Part print with two shaded views. Sizes in mm from the minimum x, y, z corner. Give positions to 0.01 mm unless a question says otherwise; leave off trailing zeros. Order: outer loops, then holes, each group sorted by start corner. A loop starts at its lowest first (then second) coordinate and runs counter-clockwise, first axis right, second up. Notation, with made-up numbers: (5, 17.25) - (14, 17.25) arc R31 cw to (14, 50.25) - close; hole circle Ø7 at (51.25, 46.5). An arc over 180 degrees is marked (long way). Return JSON: item names as keys, results as strings. Group by question number.
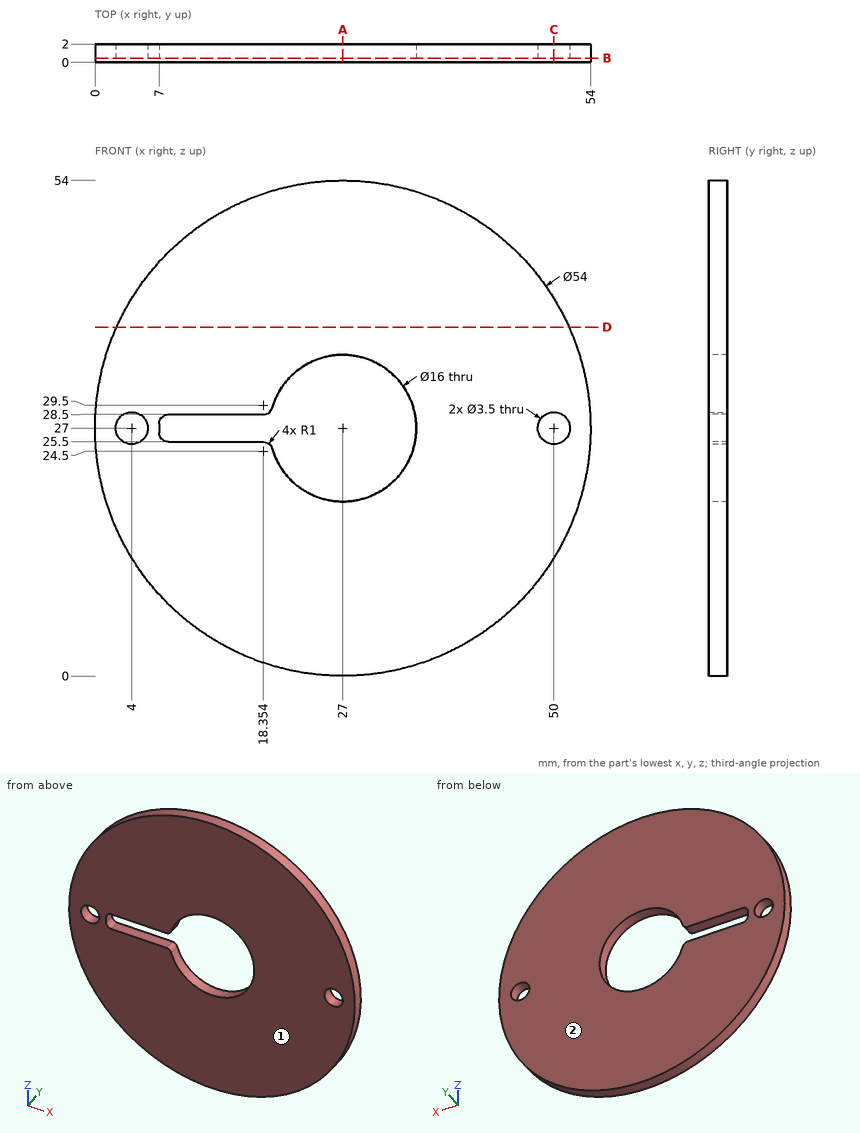
(1) Slice it at B-B (y = 0.45). State how many separate pieces and enclosed holes the cut face has, and give its area (3 significant figures).
(2) Slice it at C-C (x = 50). Give the cut face in (y, z).
(3) Slice it at A-A (x = 27). Give the cut face in (y, z).
(4) Slice it at D-D (z = 38). Give the cut face in (x, y).
(5) Drop flat-ended pins along their axis: pin 1 Ø4.5 at (x, z) = (4, 27) entering from -Y; pin 2 Ø0.6 at (x, y) = (13.5, 1.5) entering from -Z; pin 3 Ø0.5 at (y, z) = (1, 27) entering from +X. Give the stop position or say it passes through.
(6) Drill centre lines: L1, parallel to X at y = 0.8, z = 27; L2, parallel to X at y = 1.35, z = 32 (1 decimal). Where is each one in solid material? Low to high.
(7) Pull direction Y, two halves, no side cores. Call the marked faces 1 and 2: released by +Y, released by -Y, zero draft, split by the parting line, or undercut.
Result set:
{
 "1": {"separate pieces": "1", "enclosed holes": "3", "area": "2,030 mm²"},
 "2": {"outline": "(0, 12.86) - (2, 12.86) - (2, 25.25) - (0, 25.25) - close; (0, 28.75) - (2, 28.75) - (2, 41.14) - (0, 41.14) - close"},
 "3": {"outline": "(0, 0) - (2, 0) - (2, 19) - (0, 19) - close; (0, 35) - (2, 35) - (2, 54) - (0, 54) - close"},
 "4": {"outline": "(2.34, 0) - (51.66, 0) - (51.66, 2) - (2.34, 2) - close"},
 "5": {"pin 1": "stops at y = 0", "pin 2": "stops at z = 3.45", "pin 3": "stops at x = 54"},
 "6": {"L1": "x = 0 to 2.25, 5.75 to 7, 35 to 48.25, 51.75 to 54", "L2": "x = 0.5 to 20.8, 33.2 to 53.5"},
 "7": {"face 1": "released by -Y", "face 2": "released by +Y"}
}
